Work out the finished part from the listing and answer in its coordinate system (mm). A direction names the side the tool comes from. Round coordinates to 2 decimals unless told otherwise and drop trailing zeros. Loops run counter-clockwise (first coordinate to the right, second up) from the corner with the lowest first, then second, coordinate; pieces in that order, holes last.
from build123d import *

# Parameters (mm, degrees)
SKETCH_1_W          = 42
SKETCH_1_H          = 38
EXTRUDE_1_DEPTH     = 2
SKETCH_2_W          = 42
SKETCH_2_H          = 38
SKETCH_2_W_2        = 35
SKETCH_2_H_2        = 31
EXTRUDE_2_DEPTH     = 8
SKETCH_3_W          = 1
SKETCH_3_H          = 1.564579438
CUT_EXTRUDE_1_DEPTH = 6.5
CUT_EXTRUDE_3_DEPTH = 4
SKETCH_7_W          = 23
SKETCH_7_H          = 4.2
CUT_EXTRUDE_4_DEPTH = 10


with BuildPart() as part:
    # 草图1 → 凸台-拉伸1 (new body)
    with BuildSketch(Plane.XY):
        with Locations((17.5, 15.5)):
            Rectangle(SKETCH_1_W, SKETCH_1_H)
    extrude(amount=EXTRUDE_1_DEPTH)

    # 草图2 → 凸台-拉伸2 (add)
    with BuildSketch(Plane.XY.offset(2)):
        with Locations((17.5, 15.5)):
            Rectangle(SKETCH_2_W, SKETCH_2_H)
        with Locations((17.5, 15.5)):
            Rectangle(SKETCH_2_W_2, SKETCH_2_H_2, mode=Mode.SUBTRACT)
    extrude(amount=EXTRUDE_2_DEPTH)

    # 草图3 → 切除-拉伸1 (cut)
    with BuildSketch(Plane.ZY.offset(3.5)):
        Polygon((9, 31), (2, 31), (2, 24), (9, 24), (9, 29.435420562), align=None)
        with Locations((9.5, 30.217710281)):
            Rectangle(SKETCH_3_W, SKETCH_3_H)
    extrude(amount=-CUT_EXTRUDE_1_DEPTH, mode=Mode.SUBTRACT)

    # 草图6 → 切除-拉伸3 (cut)
    with BuildSketch(Plane.XY.offset(10)):
        Polygon((0, 13.5), (0, 15.5), (0, 17.5), (-3.5, 17.5), (-3.5, 13.5), align=None)
        Polygon((35, 17.5), (35, 15.5), (35, 13.5), (38.5, 13.5), (38.5, 17.5), align=None)
    extrude(amount=-CUT_EXTRUDE_3_DEPTH, mode=Mode.SUBTRACT)

    # 草图7 → 切除-拉伸4 (cut)
    with BuildSketch(Plane(origin=(0, 0, 0), x_dir=(-1, 0, 0), z_dir=(0, 0, -1))):
        with Locations((-16.5, 26)):
            Rectangle(SKETCH_7_W, SKETCH_7_H)
    extrude(amount=-CUT_EXTRUDE_4_DEPTH, mode=Mode.SUBTRACT)


solid = part.part
Item 1: Straight lines are drawn through the part: line 1 (Y direction, x = 18, z = 2.25); line 2 (X direction, y = 6, z = 4.25); line 3 (Y direction, x = -1.5, z = 7.75). For each, find the intervals that lie inside material, in ascending order.
Item 2: Each of these flat-tipped pins is pushed along its axis until it touches: P1, Ø1.8, axis at x = -1.5, y = 15.5, coming from the +Z side; P2, Ø9.5, axis at x = 21, y = 18, coming from the +Z side. Where does it stop, or does it pass through?
Item 3: Section B-B, the plane z = 8.25 is taken. Give the vertices of the cut face in (x, y), plus the area to 4 significant figures.
Item 4: For faces 5 (the face through (0, 11, 6)), 6 (the face through (5, 26, 1)), 7 (the face through (-2, 16, 6)), determine the directions among +Z, -Z, +X, -X, +Y, -Y from which every point of the face is accessible in a straight line to the end or side of a thin tool.
Item 5: Section C-C, the plane x = 11 is taken. Give the vertices of the cut face in (y, z), plus the area to 3 significant figures.
Item 6: Section A-A, the plane z = 0.75 is taken. Give the vertices of the cut face in (x, y), plus the area to 3 significant figures.
Item 7: Section D-D, the plane y = 15.5 is taken. Give the vertices of the cut face in (x, z).
Item 8: Determine the mould class of faces 1 (the face through (-1.8, 29.435, 9.5)), 2 (the face through (-2, 24, 10)), 3 (the face through (-2, 24, 5)), 4 (the face through (-2, 27, 9)) for opening direction Z: pulls with the +Z half, pulls with the -Z half, needs draft (parallel to the pull), parting line crosses it, or undercut.
Answer below:
1. line 1: y = -3.5 to 0, 31 to 34.5
1. line 2: x = -3.5 to 0, 35 to 38.5
1. line 3: y = -3.5 to 13.5, 17.5 to 24, 31 to 34.5
2. P1: stops at z = 6
2. P2: stops at z = 2
3. outline: (-3.5, -3.5) - (38.5, -3.5) - (38.5, 13.5) - (35, 13.5) - (35, 0) - (0, 0) - (0, 13.5) - (-3.5, 13.5) - close; (-3.5, 17.5) - (0, 17.5) - (0, 24) - (-3.5, 24) - close; (-3.5, 31) - (35, 31) - (35, 17.5) - (38.5, 17.5) - (38.5, 34.5) - (-3.5, 34.5) - close
3. area: 458.5 mm2
4. face 5: +Z
4. face 6: +Z, -Z
4. face 7: +Z, +X, -X
5. outline: (-3.5, 0) - (23.9, 0) - (23.9, 2) - (0, 2) - (0, 10) - (-3.5, 10) - close; (28.1, 0) - (34.5, 0) - (34.5, 10) - (31, 10) - (31, 2) - (28.1, 2) - close
5. area: 124 mm2
6. outline: (-3.5, -3.5) - (38.5, -3.5) - (38.5, 34.5) - (-3.5, 34.5) - close; hole (5, 23.9) - (28, 23.9) - (28, 28.1) - (5, 28.1) - close
6. area: 1,500 mm2
7. outline: (-3.5, 0) - (38.5, 0) - (38.5, 6) - (35, 6) - (35, 2) - (0, 2) - (0, 6) - (-3.5, 6) - close
8. face 1: needs draft
8. face 2: pulls with the +Z half
8. face 3: undercut
8. face 4: undercut
